Geometry check sheet. Reference: the model listing, model coordinates, mm. A direction names the side the tool comes from. Give positions to 0.01 mm unless a question says otherwise; leave off trailing zeros. Loops run counter-clockwise (first coordinate to the right, second up) from the corner with the lowest first, then second, coordinate; pieces in that order, holes last.
1. Material ranges on L1, parallel to Y at x = 110.5, z = 6.75; L2, parallel to X at y = 150, z = 11.25; L3, parallel to X at y = 202.5, z = 12.5, recorded low to high.
2. Cross-section at A-A, the plane z = 8.75. Record the cut outline in (x, y).
3. Tool access check on faces 1 (the cylindrical face through (2.406, 2.281, 8.381)), 2 (the cylindrical face through (7.406, 109.06, 17.719)). Record the directions out of +Z, -Z, +X, -X, +Y, -Y that give a thin tool (end or side, any length) a straight path to the whole face; none if there is none.
4. Cross-section at C-C, the plane y = 67. Record the cut outline in (x, z).
5. Cross-section at B-B, the plane x = 111.5. Record the cut outline in (y, z), plus the area to 3 significant figures.
6. Go/stop test with flat-tipped pins: pin 1 Ø8 at (x, y) = (14, 97) entering from -Z; pin 2 Ø2 at (y, z) = (186.5, 18.5) entering from +X; pin 3 Ø1 at (x, y) = (41, 83) entering from -Z. Record where each tip stops, or that it passes through.
7. Release check for a two-part mould opening along X. For faces 3 (the flat face through (69, 220.849, 8)), 4 (the flat face through (135.651, 109, 8)), 5 (the flat face through (67, 215.849, 6)) record: +X half, -X half, draft (parallel to the pull), parting line (faces both ways), or undercut.
Autodesk Inventor part; units mm, degrees
ref_plane "YZ Plane" through (0, 0, 0) normal (1, 0, 0) x (0, 1, 0)
ref_plane "XZ Plane" through (0, 0, 0) normal (0, 1, 0) x (-1, 0, 0)
ref_plane "XY Plane" through (0, 0, 0) normal (0, 0, 1) x (1, 0, 0)
sketch "Эскиз1" plane through (0, 0, 0) normal (0, 0, 1) x (1, 0, 0)
  line L0 (5, 13) -> (5, 207.8488)
  arc A0 (13, 215.8488) -> (5, 207.8488) centre (13, 207.8488) ccw
  line L1 (13, 215.8488) -> (122.6512, 215.8488)
  arc A1 (130.6512, 207.8488) -> (122.6512, 215.8488) centre (122.6512, 207.8488) ccw
  line L2 (130.6512, 207.8488) -> (130.6512, 13)
  arc A2 (122.6512, 5) -> (130.6512, 13) centre (122.6512, 13) ccw
  line L3 (13, 5) -> (122.6512, 5)
  arc A3 (5, 13) -> (13, 5) centre (13, 13) ccw
  arc A4 (127.6512, 0) -> (135.6512, 8) centre (127.6512, 8) ccw
  line L4 (135.6512, 8) -> (135.6512, 212.8488)
  arc A5 (135.6512, 212.8488) -> (127.6512, 220.8488) centre (127.6512, 212.8488) ccw
  line L5 (127.6512, 220.8488) -> (8, 220.8488)
  arc A6 (8, 220.8488) -> (0, 212.8488) centre (8, 212.8488) ccw
  line L6 (0, 8) -> (0, 212.8488)
  arc A7 (0, 8) -> (8, 0) centre (8, 8) ccw
  line L7 (127.6512, 0) -> (8, 0)
  point P0 (0, 0)
extrude "Выдавливание1" add sketch "Эскиз1" along normal blind 20
sketch "Эскиз2" plane through (0, 0, 20) normal (0, 0, 1) x (1, 0, 0)
  line L0 (8, 0) -> (127.6512, 0)
  arc A0 (127.6512, 0) -> (135.6512, 8) centre (127.6512, 8) ccw
  line L1 (135.6512, 8) -> (135.6512, 212.8488)
  arc A1 (135.6512, 212.8488) -> (127.6512, 220.8488) centre (127.6512, 212.8488) ccw
  line L2 (127.6512, 220.8488) -> (8, 220.8488)
  arc A2 (8, 220.8488) -> (0, 212.8488) centre (8, 212.8488) ccw
  line L3 (0, 212.8488) -> (0, 8)
  arc A3 (0, 8) -> (8, 0) centre (8, 8) ccw
  arc A4 (5, 13) -> (13, 5) centre (13, 13) ccw
  line L4 (5, 13) -> (5, 207.8488)
  arc A5 (13, 215.8488) -> (5, 207.8488) centre (13, 207.8488) ccw
  line L5 (13, 215.8488) -> (122.6512, 215.8488)
  arc A6 (130.6512, 207.8488) -> (122.6512, 215.8488) centre (122.6512, 207.8488) ccw
  line L6 (130.6512, 207.8488) -> (130.6512, 13)
  arc A7 (122.6512, 5) -> (130.6512, 13) centre (122.6512, 13) ccw
  line L7 (122.6512, 5) -> (13, 5)
  point P0 (0, 0)
extrude "Выдавливание2" add sketch "Эскиз2" along normal blind 5 contours A3 L3 A2 L2 A1 L1 A0 L0 | L4 A5 L5 A6 L6 A7 L7 A4
fillet "Сопряжение1" radius 8 16 edges at (133.308, 218.5056, 25) (67.8256, 220.8488, 25) (2.3431, 218.5056, 25) (0, 110.4244, 25) (2.3431, 2.3431, 25) (67.8256, 0, 25) (133.308, 2.3431, 25) (135.6512, 110.4244, 25) (128.308, 7.3431, 20) (67.8256, 5, 20) (7.3431, 7.3431, 20) (5, 110.4244, 20) (7.3431, 213.5056, 20) (67.8256, 215.8488, 20) (128.308, 213.5056, 20) (130.6512, 110.4244, 20)
properties part number "kris"
Result:
1. L1: y = 0 to 5, 215.85 to 220.85
1. L2: x = 0 to 5, 130.65 to 135.65
1. L3: x = 0 to 5.02, 130.64 to 135.65
2. outline: (0, 8) arc R8 ccw to (8, 0) - (127.65, 0) arc R8 ccw to (135.65, 8) - (135.65, 212.85) arc R8 ccw to (127.65, 220.85) - (8, 220.85) arc R8 ccw to (0, 212.85) - close; hole (5, 13) arc R8 ccw to (13, 5) - (122.65, 5) arc R8 ccw to (130.65, 13) - (130.65, 207.85) arc R8 ccw to (122.65, 215.85) - (13, 215.85) arc R8 ccw to (5, 207.85) - close
3. face 1: +Z, -Z, -X, -Y
3. face 2: -Z
4. outline: (0, 0) - (5, 0) - (5, 12) arc R8 cw to (13, 20) - (122.65, 20) arc R8 cw to (130.65, 12) - (130.65, 0) - (135.65, 0) - (135.65, 17) arc R8 ccw to (127.65, 25) - (8, 25) arc R8 ccw to (0, 17) - close
5. outline: (0, 0) - (5, 0) - (5, 12) arc R8 cw to (13, 20) - (207.85, 20) arc R8 cw to (215.85, 12) - (215.85, 0) - (220.85, 0) - (220.85, 17) arc R8 ccw to (212.85, 25) - (8, 25) arc R8 ccw to (0, 17) - close
5. area: 1,300 mm2
6. pin 1: stops at z = 19.42
6. pin 2: stops at x = 135.64
6. pin 3: stops at z = 20
7. face 3: draft
7. face 4: +X half
7. face 5: undercut
